Build history of the part. All positions in model axes, mm. Coordinates: 2 decimals unless noted, no trailing zeros. Order: outer loops, then holes, each group sorted by start corner. A loop starts at its lowest first (then second) coordinate and runs counter-clockwise, first axis right, second up. Notation, with made-up numbers: (-10, -28.5) - (41, -28.5) arc R13 ccw to (41, -13.5) - close; hole circle Ø10 at (67.5, 23.5). An arc over 180 degrees is marked (long way). One line per item, written item: value.
from build123d import *

# Parameters (mm, degrees)
ESBO_O1_R                = 7.5
ESBO_O1_R_2              = 5.05
RESSALTO_EXTRUS_O1_DEPTH = 7.25
CHANFRO1_SIZE            = 0.5


with BuildPart() as part:
    # Esboço1 → Ressalto-extrusão1 (new, symmetric)
    with BuildSketch(Plane.XY):
        with Locations(Location((0, 0, 0), (0, 0, 180))):
            Circle(ESBO_O1_R)
        with Locations(Location((0, 0, 0), (0, 0, 180))):
            Circle(ESBO_O1_R_2, mode=Mode.SUBTRACT)
    extrude(amount=RESSALTO_EXTRUS_O1_DEPTH, both=True)

    # Chanfro1
    chanfro1_edges = [part.edges().sort_by_distance(p)[0] for p in [
        (7.5, 0, -7.25),
        (7.5, 0, 7.25),
        (5.05, 0, -7.25),
        (5.05, 0, 7.25),
    ]]
    chamfer(chanfro1_edges, length=CHANFRO1_SIZE)


solid = part.part
1. Probe line 1 along Y through (x, z) = (0, 2); line 2 along Z through (x, y) = (5.25, -0.75); line 3 along X through (y, z) = (-3.25, -4). List the from-to ranges inside material, lowest first.
Values found:
line 1: y = -7.5 to -5.05, 5.05 to 7.5
line 2: z = -7 to 7
line 3: x = -6.76 to -3.87, 3.87 to 6.76
2. Flat gauge pins, fed straight in: P1, Ø2, axis at y = 2.5, z = -3, coming from the +X side; P2, Ø8, axis at x = 3.5, y = -3, coming from the +Z side; P3, Ø1, axis at x = -5, y = -0.5, coming from the -Z side; P4, Ø5, axis at y = 3.5, z = -5, coming from the +X side. Where does each tip first touch, or does it go through?
Values found:
P1: stops at x = 7.35
P2: stops at z = 7.25
P3: stops at z = -7.22
P4: stops at x = 7.43
3. Band-saw the part on C-C, the plane z = 2.5. Give the cut face in (x, y).
Values found:
outline: circle Ø15 at (0, 0); hole circle Ø10.1 at (0, 0)
4. Two-plate mould, pull along X, no slides. Class faces 1 (the face through (-4.032, -6.324, 0.095)), 2 (the face through (5, -3, 7.25)), 3 (the face through (4.01, 3.07, -0.09)): pulls with the +X half, pulls with the -X half, needs draft (parallel to the pull), parting line crosses it, or undercut.
Values found:
face 1: parting line crosses it
face 2: needs draft
face 3: undercut
5. Band-saw the part on A-A, the plane x = 0. Give the cut face in (y, z), and give its area (4 significant figures).
Values found:
outline: (-7.5, -6.75) - (-7, -7.25) - (-5.55, -7.25) - (-5.05, -6.75) - (-5.05, 6.75) - (-5.55, 7.25) - (-7, 7.25) - (-7.5, 6.75) - close; (5.05, -6.75) - (5.55, -7.25) - (7, -7.25) - (7.5, -6.75) - (7.5, 6.75) - (7, 7.25) - (5.55, 7.25) - (5.05, 6.75) - close
area: 70.05 mm2
